Here's how the part is built. I have some questions about the finished solid (model axes, mm). A direction names the side the tool comes from. Give positions to 0.01 mm unless a question says otherwise; leave off trailing zeros. Order: outer loops, then holes, each group sorted by start corner. A loop starts at its lowest first (then second) coordinate and runs counter-clockwise, first axis right, second up. Notation, with made-up numbers: (10.5, 37.25) -> (34.5, 37.25) arc R24 cw to (34.5, 71.25) -> close; hole circle Ø3 at (-9.75, 51.25). An arc over 180 degrees is marked (long way). Write each question's results on one line, items separated by ' | '. Start each with the question number.
Q1. For faces 1 (the face through (13.29, -12.52, 10.49)), 2 (the face through (-2.001, -12.522, 103.173)), which set-ups out of +Z, -Z, +X, -X, +Y, -Y let a thin tool reach every point of the face, with its end or its side?
Q2. I'm going to push flat-ended pins straight in: pin 1 (10 mm diameter, centred on x = 6, y = -17, fed in from -Z); pin 2 (8 mm diameter, centred on y = -16, z = 44.5, fed in from +X); pin 3 (2 mm diameter, centred on y = -10, z = 14, fed in from -X). Where does each tip first touch, or does it pass through?
Q3. I need wall thicknesses on line 1 along Z through (x, y) = (44.45, -6) (1 decimal); line 2 along Z through (x, y) = (-0.5, -9); line 3 along Z through (x, y) = (42.5, -14.75). Which ranges of each line are inside material? Lowest first, please. Write a range as [from, to].
Q4. Imagine slicing it at C-C, the plane z = 79.5. Please give me the cut outline in (x, y).
Q5. Imagine slicing it at B-B, the plane x = 39. Please give me the cut outline in (y, z).
Q6. Thinking about a two-plate mould opening in Z: for faces 3 (the face through (32, -13, 7.938)), 4 (the face through (-15.873, -12.522, 63.731)), 5 (the face through (13.473, -12.522, 38.978)), which applies, pulls with the +Z half, pulls with the -Z half, needs draft (parallel to the pull), parting line crosses it, or undercut?
Q7. Imagine slicing it at A-A, the plane y = -4.5. State how many separate pieces and enclosed holes the cut face has, then the cut area to 3 significant figures.
```python
from build123d import *

# Parameters (mm, degrees)
F0_R     = 3.175
F1_DEPTH = 25.4


with BuildPart() as f1:
    # F0 (on Front) → F1 (new body)
    with BuildSketch(Plane.XZ):
        with BuildLine():
            ThreePointArc((-9.525, 114.3), (0, 104.775), (9.525, 114.3))
            ThreePointArc((9.525, 114.3), (0, 123.825), (-9.525, 114.3))
        make_face()
        with Locations((0, 114.3)):
            Circle(F0_R, mode=Mode.SUBTRACT)
        with BuildLine():
            Line((14.971058, 68.780441), (9.525, 114.3))
            ThreePointArc((9.525, 114.3), (0, 104.775), (-9.525, 114.3))
            Line((-9.525, 114.3), (-15.747457, 65.508289))
            ThreePointArc((-15.747457, 65.508289), (-1.6815, 79.285695), (14.971058, 68.780441))
        make_face()
        with Locations((-1.5875, 100.0252)):
            Circle(F0_R, mode=Mode.SUBTRACT)
        with BuildLine():
            Line((15.794203, 61.90038), (14.971058, 68.780441))
            ThreePointArc((14.971058, 68.780441), (-1.6815, 79.285695), (-15.747457, 65.508289))
            ThreePointArc((-15.747457, 65.508289), (-15.873668, 63.705667), (-15.794203, 61.90038))
            ThreePointArc((-15.794203, 61.90038), (0, 47.625), (15.794203, 61.90038))
        make_face()
        with Locations((0, 63.5)):
            Circle(F0_R, mode=Mode.SUBTRACT)
        with BuildLine():
            ThreePointArc((15.875, 63.5), (15.647383, 66.178627), (14.971058, 68.780441))
            Line((14.971058, 68.780441), (15.794203, 61.90038))
            ThreePointArc((15.794203, 61.90038), (15.854788, 62.699171), (15.875, 63.5))
        make_face()
        with BuildLine():
            Line((11.215222, 16.688789), (15.794203, 61.90038))
            ThreePointArc((15.794203, 61.90038), (0, 47.625), (-15.794203, 61.90038))
            Line((-15.794203, 61.90038), (-9.525, 0))
            ThreePointArc((-9.525, 0), (-6.735192, 6.735192), (0, 9.525))
            ThreePointArc((0, 9.525), (0.338886, 9.51897), (0.677344, 9.500886))
            ThreePointArc((0.677344, 9.500886), (6.970557, 6.491299), (9.525, 0))
            ThreePointArc((9.525, 0), (6.970557, -6.491299), (0.677344, -9.500886))
            Line((0.677344, -9.500886), (44.732405, -7.932475))
            ThreePointArc((44.732405, -7.932475), (36.513756, -0.141225), (44.45, 7.9375))
            Line((44.45, 7.9375), (19.124959, 7.9375))
            ThreePointArc((19.124959, 7.9375), (13.226887, 10.556806), (11.215222, 16.688789))
        make_face()
        with BuildLine():
            ThreePointArc((0, 9.525), (-6.735192, 6.735192), (-9.525, 0))
            ThreePointArc((-9.525, 0), (-6.735192, -6.735192), (0, -9.525))
            Line((0, -9.525), (0.677344, -9.500886))
            ThreePointArc((0.677344, -9.500886), (6.970557, -6.491299), (9.525, 0))
            ThreePointArc((9.525, 0), (6.970557, 6.491299), (0.677344, 9.500886))
            Line((0.677344, 9.500886), (0, 9.525))
        make_face()
        Circle(F0_R, mode=Mode.SUBTRACT)
        with BuildLine():
            Line((0.677344, -9.500886), (0, -9.525))
            ThreePointArc((0, -9.525), (0.338886, -9.51897), (0.677344, -9.500886))
        make_face()
        with BuildLine():
            ThreePointArc((52.3875, 0), (50.06266, 5.61266), (44.45, 7.9375))
            ThreePointArc((44.45, 7.9375), (36.513756, -0.141225), (44.732405, -7.932475))
            ThreePointArc((44.732405, -7.932475), (50.161633, -5.51191), (52.3875, 0))
        make_face()
        with Locations((44.45, 0)):
            Circle(F0_R, mode=Mode.SUBTRACT)
    extrude(amount=F1_DEPTH)


solid = f1.part
```
Geometry check:
1) face 1: +X, +Y, -Y | face 2: +Y, -Y
2) pin 1: z = -9.49 | pin 2: x = 14.44 | pin 3: x = -11.04
3) line 1: [-7.9, -3.2], [3.2, 7.9] | line 2: [-9.51, -3.14], [3.14, 60.36], [66.64, 97.04], [103.01, 111.16], [117.44, 123.81] | line 3: [-8.01, -2.51], [2.51, 7.94]
4) outline: (-13.96, -25.4) -> (13.69, -25.4) -> (13.69, 0) -> (-13.96, 0) -> close
5) outline: (-25.4, -8.14) -> (0, -8.14) -> (0, 7.94) -> (-25.4, 7.94) -> close
6) face 3: pulls with the +Z half | face 4: parting line crosses it | face 5: undercut
7) separate pieces: 1 | enclosed holes: 6 | area: 3,740 mm²
